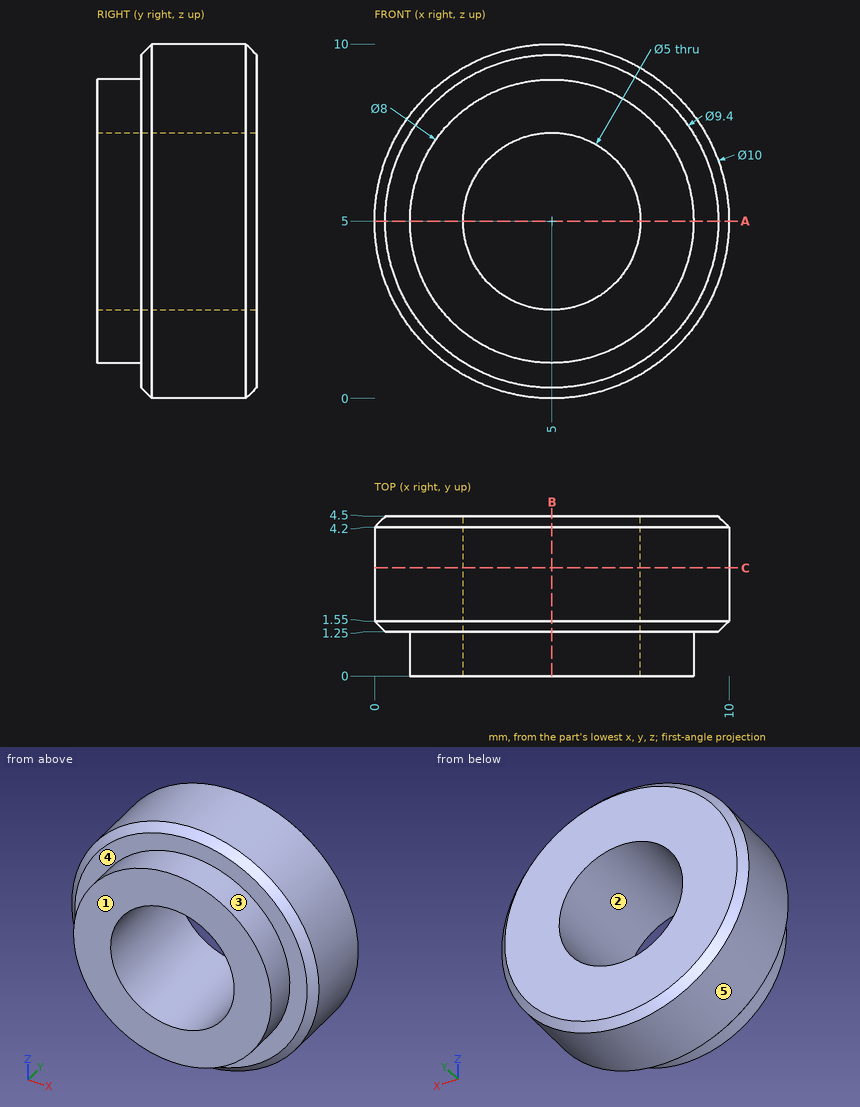
For this review, use the dimensioned drawing (mm, ordinates from the lowest corner) and the shaded views. A direction names the side the tool comes from. Give positions to 0.01 mm unless a question says otherwise; leave off trailing zeros. Loops run counter-clockwise (first coordinate to the right, second up) from the corner with the lowest first, then second, coordinate; pieces in that order, holes last. Notation, with made-up numbers: (-25, 74.25) -> (32, 74.25) arc R27 ccw to (32, 96.25) -> close; hole circle Ø10 at (87.5, 43). An arc over 180 degrees is marked (long way). Use CSV: the item, a comma, the result in double quotes.
1. Machinability: for the marked faces 4 and 5, which of the approach directions +Z, -Z, +X, -X, +Y, -Y give a long, thin tool a straight path to every point of the face, cutting with its end or side? Answer none if there is none.
Result:
face 4,"-Y"
face 5,"+Y, -Y"
2. For P1, Ø3, axis at x = 5, z = 5, coming from the -Y side; P2, Ø1, axis at y = 1.5, z = 5.5, coming from the -X side; P3, Ø2, axis at x = 1.5, y = 2.5, coming from the -Z side, all flat-tipped, find the tip position at first contact; note any pin that passes through.
Result:
P1,"passes through"
P2,"stops at x = 0"
P3,"stops at z = 0.67"
3. To check wall thickness, follow probe 1 along X at (y, z) = (1.15, 5); probe 2 along X at (y, z) = (2.3, 5); probe 3 along Y at (x, z) = (4.5, 9.5). State the ranges of each line that lie inside material, in increasing order. Write a range as from..to.
Result:
probe 1,"x = 1..2.5, 7.5..9"
probe 2,"x = 0..2.5, 7.5..10"
probe 3,"y = 1.25..4.5"
4. Consider section B-B, the plane x = 5. Write out the cut boundary in (y, z).
Result:
outline,"(0, 1) -> (1.25, 1) -> (1.25, 0.3) -> (1.55, 0) -> (4.2, 0) -> (4.5, 0.3) -> (4.5, 2.5) -> (0, 2.5) -> close; (0, 7.5) -> (4.5, 7.5) -> (4.5, 9.7) -> (4.2, 10) -> (1.55, 10) -> (1.25, 9.7) -> (1.25, 9) -> (0, 9) -> close"
5. The part is to be moulded in two halves that separate along X. For the marked faces 1, 2 and 3, say which applies: +X half, -X half, draft (parallel to the pull), parting line (faces both ways), or undercut.
Result:
face 1,"draft"
face 2,"undercut"
face 3,"parting line"
6. Consider section A-A, the plane z = 5. Write out the cut boundary in (x, y).
Result:
outline,"(0, 1.55) -> (0.3, 1.25) -> (1, 1.25) -> (1, 0) -> (2.5, 0) -> (2.5, 4.5) -> (0.3, 4.5) -> (0, 4.2) -> close; (7.5, 0) -> (9, 0) -> (9, 1.25) -> (9.7, 1.25) -> (10, 1.55) -> (10, 4.2) -> (9.7, 4.5) -> (7.5, 4.5) -> close"
7. Consider section C-C, the plane y = 3.05. Write out the cut boundary in (x, z).
Result:
outline,"circle Ø10 at (5, 5); hole circle Ø5 at (5, 5)"
